Verification items for this drawing (mm, ordinates from the low corner). A direction names the side the tool comes from. Coordinates: 2 decimals unless noted, no trailing zeros. Write each loop counter-clockwise with the first axis right and the second up, starting at its lowest first coordinate (ties: lowest second). Pieces come first, ordered by that corner, then holes. Notation, with made-up numbers: M 61,59.25 L 114,59.25 A11 ccw 114,68.25 Z; hole C 82.5,49 d7. An arc over 180 degrees is marked long. Put each result on its own line as item: value. Start each with the question number.
1) Cross-section at D-D on z = 18. Record the cut outline in (x, y), plus the area to 3 significant figures.
2) Cross-section at C-C on y = 26. Record the cut outline in (x, z).
3) Cross-section at A-A on z = 10. Record the cut outline in (x, y).
4) Mould release check, pull along X, two halves, no side actions. Record for the marked faces 4, 5 and 6: released by +X, released by -X, zero draft, split by the parting line, or undercut.
5) Cross-section at B-B on x = 22.5. Record the cut outline in (y, z), plus the area to 3 significant figures.
6) Set-up check for the marked faces 1, 2 and 3: record each of +Z, -Z, +X, -X, +Y, -Y from which the full face is reachable in a straight line by a thin tool's end or side.
7) Gauge pin test, flat ends, axial feed: pin 1 (9 mm diameter, centred on y = 14, z = 14.5, fed in from +X); pin 2 (2 mm diameter, centred on x = 16, z = 11.5, fed in from -Y); pin 3 (6 mm diameter, centred on x = 9.5, z = 15, fed in from +Y); pin 4 (11 mm diameter, centred on x = 5.5, z = 15, fed in from +Y). Record the tip position at first contact, or that the pin passes through.
8) Scan lines: line 1 along X through (y, z) = (2.75, 10); line 2 along Y through (x, z) = (7, 16.5); line 3 along Y through (x, z) = (28, 13.5). Record each from-to range of solid material in increasing order.
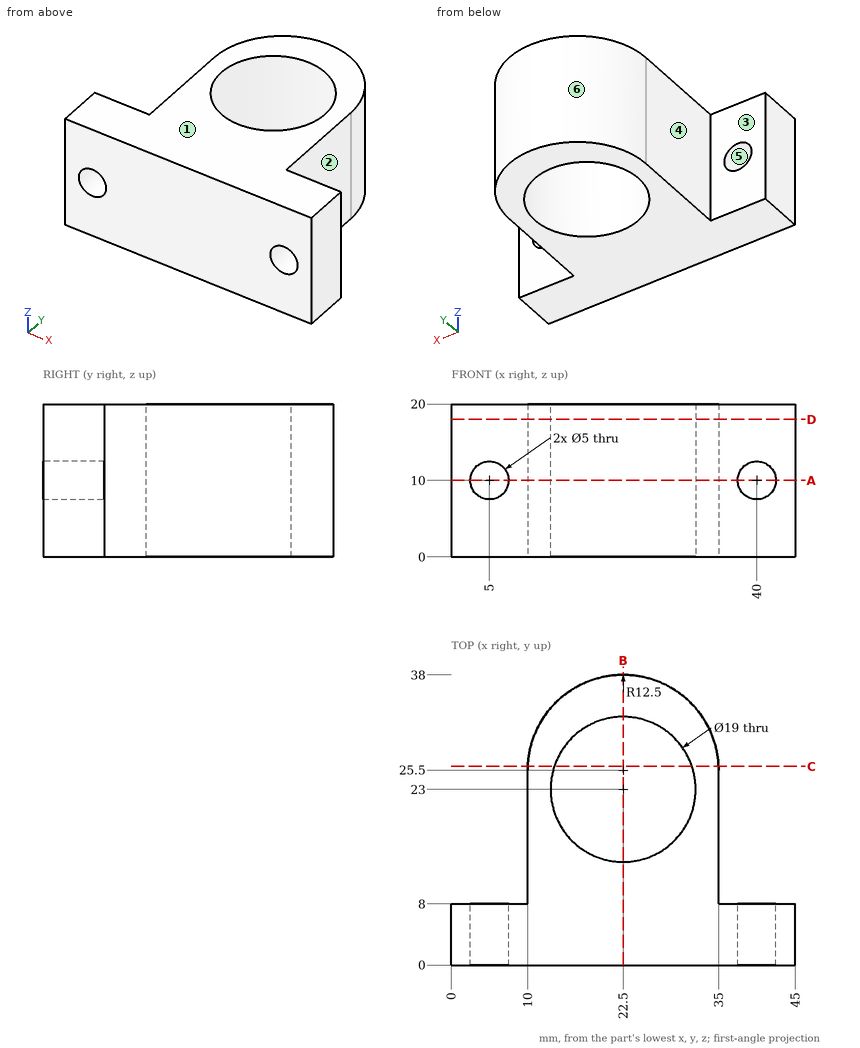
Answer key:
1. outline: M 0,0 L 45,0 L 45,8 L 35,8 L 35,25.5 A12.5 ccw 10,25.5 L 10,8 L 0,8 Z; hole C 22.5,23 d19
1. area: 759 mm²
2. outline: M 10.01,0 L 13.49,0 L 13.49,20 L 10.01,20 Z; M 31.51,0 L 34.99,0 L 34.99,20 L 31.51,20 Z
3. outline: M 0,0 L 2.5,0 L 2.5,8 L 0,8 Z; M 7.5,0 L 37.5,0 L 37.5,8 L 35,8 L 35,25.5 A12.5 ccw 10,25.5 L 10,8 L 7.5,8 Z; M 42.5,0 L 45,0 L 45,8 L 42.5,8 Z; hole C 22.5,23 d19
4. face 4: released by -X
4. face 5: undercut
4. face 6: split by the parting line
5. outline: M 0,0 L 13.5,0 L 13.5,20 L 0,20 Z; M 32.5,0 L 38,0 L 38,20 L 32.5,20 Z
5. area: 380 mm²
6. face 1: +Z, +X, -X, +Y, -Y
6. face 2: +Z, -Z, +X, +Y
6. face 3: +Z, -Z, -X, +Y
7. pin 1: stops at x = 35
7. pin 2: stops at y = 0
7. pin 3: stops at y = 33
7. pin 4: stops at y = 30.4
8. line 1: x = 0 to 2.5, 7.5 to 37.5, 42.5 to 45
8. line 2: y = 0 to 8
8. line 3: y = 0 to 15.25, 30.75 to 36.72
